from build123d import *

# Parameters (mm, degrees)
SKETCH1_W            = 12.7
SKETCH1_H            = 6.35
SKETCH1_W_2          = 9.525
SKETCH1_H_2          = 3.175
BOSS_EXTRUDE1_DEPTH  = 355.6
CUT_EXTRUDE1_DEPTH   = 25.4
LPATTERN1_COUNT      = 2
LPATTERN1_PITCH      = 57.15
MIRROR1_COPY_1_DEPTH = 25.4
SKETCH3_W            = 12.7
SKETCH3_H            = 3.175
CUT_EXTRUDE2_DEPTH   = 25.4
SKETCH4_R            = 2.0955
CUT_EXTRUDE3_DEPTH   = 25.4


with BuildPart() as part:
    # Sketch1 → Boss-Extrude1 (new body)
    with BuildSketch(Plane.XY):
        Rectangle(SKETCH1_W, SKETCH1_H)
        Rectangle(SKETCH1_W_2, SKETCH1_H_2, mode=Mode.SUBTRACT)
    extrude(amount=BOSS_EXTRUDE1_DEPTH)

    # Sketch2 → Cut-Extrude1 (cut)
    with BuildSketch(Plane(origin=(0, 3.175, 0), x_dir=(1, 0, 0), z_dir=(0, 1, 0))):
        with BuildLine():
            Line((-3.175, -209.55), (-3.175, -252.73))
            ThreePointArc((-3.175, -252.73), (0, -255.905), (3.175, -252.73))
            Line((3.175, -252.73), (3.175, -209.55))
            ThreePointArc((3.175, -209.55), (0, -206.375), (-3.175, -209.55))
        make_face()
    cut_extrude1 = extrude(amount=-CUT_EXTRUDE1_DEPTH, mode=Mode.SUBTRACT)

    # LPattern1: Cut-Extrude1 ×2
    with Locations(*[(0, 0, i * LPATTERN1_PITCH) for i in range(1, LPATTERN1_COUNT)]):
        add(cut_extrude1, mode=Mode.SUBTRACT)

    # Mirror1: Cut-Extrude1 across plane
    add(cut_extrude1.mirror(Plane.XY.offset(177.8)), mode=Mode.SUBTRACT)

    # Mirror1 copy 1 sketch → Mirror1 copy 1 (cut)
    with BuildSketch(Plane(origin=(0, 3.175, 298.45), x_dir=(1, 0, 0), z_dir=(0, 1, 0))):
        with BuildLine():
            Line((-3.175, 209.55), (-3.175, 252.73))
            ThreePointArc((-3.175, 252.73), (0, 255.905), (3.175, 252.73))
            Line((3.175, 252.73), (3.175, 209.55))
            ThreePointArc((3.175, 209.55), (0, 206.375), (-3.175, 209.55))
        make_face()
    extrude(amount=-MIRROR1_COPY_1_DEPTH, mode=Mode.SUBTRACT)

    # Sketch3 → Cut-Extrude2 (cut)
    with BuildSketch(Plane(origin=(6.35, 0, 0), x_dir=(0, 0, -1), z_dir=(1, 0, 0))):
        with Locations((-177.8, 1.5875)):
            Rectangle(SKETCH3_W, SKETCH3_H)
    extrude(amount=-CUT_EXTRUDE2_DEPTH, mode=Mode.SUBTRACT)

    # Sketch4 → Cut-Extrude3 (cut)
    with BuildSketch(Plane(origin=(0, -3.175, 0), x_dir=(-1, 0, 0), z_dir=(0, -1, 0))):
        with Locations(Location((0, -177.8, 0), (0, 0, 90))):
            Circle(SKETCH4_R)
        with Locations(Location((0, -196.85, 0), (0, 0, 90))):
            Circle(SKETCH4_R)
        with Locations(Location((0, -158.75, 0), (0, 0, 270))):
            Circle(SKETCH4_R)
    extrude(amount=-CUT_EXTRUDE3_DEPTH, mode=Mode.SUBTRACT)


solid = part.part
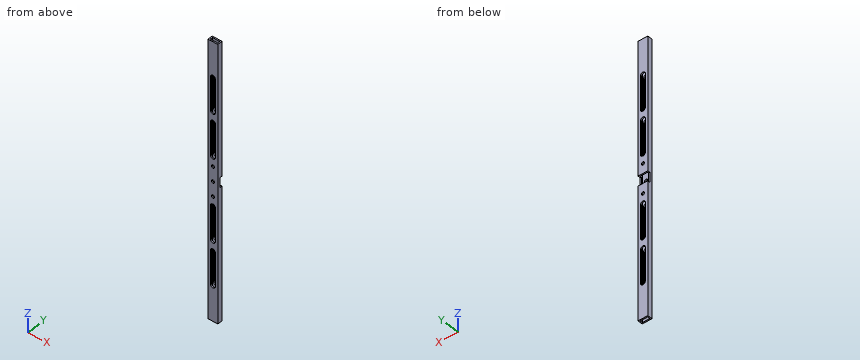
Input: part model. Units: mm. Frame: model coordinates. Coordinates: 2 decimals unless noted, no trailing zeros. Write each question's results on one line, items separated by ' | '. Start each with the question number.
Q1. Ray query, line 1 (Y direction, x = 4.5, z = 219.5) (1 decimal); line 2 (Z direction, x = 4.5, y = 2); line 3 (X direction, y = 2.4, z = 196.85). Return the intervals inside material, ascending. Write a range as from..to.
Q2. Section B-B, the plane x = 0. State how many separate pieces and enclosed holes the cut face has, plus the area to 3 significant figures.
Q3. Pin query (flat end, axial travel): pin 1 (6.5 mm diameter, centred on x = 0, z = 196.85, fed in from +Y) (3 decimals); pin 2 (0.8 mm diameter, centred on x = 5.5, z = 175.5, fed in from +Y). Return the tip coordinate at first contact, or that it passes through.
Found:
1) line 1: -3.2..-1.6, 1.6..3.2 | line 2: 0..171.45, 184.15..355.6 | line 3: -6.35..-2.1, 2.1..6.35
2) separate pieces: 16 | enclosed holes: 0 | area: 447 mm2
3) pin 1: y = 3.175 | pin 2: y = 0
